from build123d import *

# Parameters (mm, degrees)
F0_R     = 12.5
F1_DEPTH = 25
F2_R     = 7.5
F3_DEPTH = 18
F4_R     = 6.85
F5_DEPTH = 7
F7_DEPTH = 13
F8_SIZE  = 0.5


with BuildPart() as f1:
    # F0 (on Top) → F1 (new body)
    with BuildSketch(Plane.XY):
        Circle(F0_R)
    extrude(amount=F1_DEPTH)

    # F2 (on face) → F3 (cut)
    with BuildSketch(Plane(origin=(0, 0, 0), x_dir=(1, 0, 0), z_dir=(0, 0, -1))):
        Circle(F2_R)
    extrude(amount=-F3_DEPTH, mode=Mode.SUBTRACT)

    # F4 (on face) → F5 (cut)
    with BuildSketch(Plane.XY.offset(25)):
        Circle(F4_R)
    extrude(amount=-F5_DEPTH, mode=Mode.SUBTRACT)

    # F6 (on face) → F7 (cut)
    with BuildSketch(Plane.XY.offset(25)):
        with BuildLine():
            ThreePointArc((-5.9371710435, -11), (-3.0618621785, -12.1191996435), (0, -12.5))
            Line((0, -12.5), (0, -11))
            Line((0, -11), (-5.9371710435, -11))
        make_face()
        with BuildLine():
            Line((0, -11), (0, -12.5))
            ThreePointArc((0, -12.5), (3.0618621785, -12.1191996435), (5.9371710435, -11))
            Line((5.9371710435, -11), (0, -11))
        make_face()
    extrude(amount=-F7_DEPTH, mode=Mode.SUBTRACT)

    # F8
    f8_edges = [f1.edges().sort_by_distance(p)[0] for p in [
        (-12.5, 0, 0),
    ]]
    chamfer(f8_edges, length=F8_SIZE)


solid = f1.part
Can you work these out from the model? Positions are in its coordinate system, mm. A direction names the side the tool comes from. Give positions to 0.01 mm unless a question says otherwise; leave off trailing zeros. Loops run counter-clockwise (first coordinate to the right, second up) from the corner with the lowest first, then second, coordinate; pieces in that order, holes last. Notation, with made-up numbers: (73.25, 8.5) - (96.25, 8.5) arc R9 cw to (96.25, 25.5) - close; hole circle Ø5 at (76, 14.25). An arc over 180 degrees is marked (long way). Return JSON: item names as keys, results as strings.
1. If I drill on line 1 (Y direction, x = 0, z = 21); line 2 (Y direction, x = 0, z = 8.75), over which ranges is the centre line in solid material (lowest first)?
Output values:
{"line 1": "y = -11 to -6.85, 6.85 to 12.5", "line 2": "y = -12.5 to -7.5, 7.5 to 12.5"}
2. For faces 1 (the face through (-6, -5, 0)), 2 (the face through (0, -12, 12)), 3 (the face through (-7.493, -0.33, 8.874)), which set-ups out of +Z, -Z, +X, -X, +Y, -Y let a thin tool reach every point of the face, with its end or its side?
Output values:
{"face 1": "-Z, +X, -X, +Y, -Y", "face 2": "+Z, +X, -X, -Y", "face 3": "-Z"}
3. I'm going to push flat-ended pins straight in: pin 1 Ø10 at (x, z) = (6.5, 21) entering from -Y; pin 2 Ø10 at (x, z) = (-6, 20) entering from +Y; pin 3 Ø4 at (y, z) = (6.5, 11) entering from +X; pin 4 Ø1.5 at (x, y) = (1, 4.5) entering from -Z. Where does each tip first touch, or does it pass through?
Output values:
{"pin 1": "stops at y = -11", "pin 2": "stops at y = 12.46", "pin 3": "stops at x = 11.66", "pin 4": "passes through"}
4. I want a section at D-D on z = 14.5. Please give me the cut outline in (x, y).
Output values:
{"outline": "(-5.94, -11) - (5.94, -11) arc R12.5 ccw (long way) to start; hole circle Ø15 at (0, 0)"}
5. I want a section at B-B on x = 0. Please give me the cut outline in (y, z).
Output values:
{"outline": "(-12.5, 0.5) - (-12, 0) - (-7.5, 0) - (-7.5, 18) - (-6.85, 18) - (-6.85, 25) - (-11, 25) - (-11, 12) - (-12.5, 12) - close; (6.85, 18) - (7.5, 18) - (7.5, 0) - (12, 0) - (12.5, 0.5) - (12.5, 25) - (6.85, 25) - close"}
6. I want a section at C-C on z = 7.5. Please give me the cut outline in (x, y).
Output values:
{"outline": "circle Ø25 at (0, 0); hole circle Ø15 at (0, 0)"}
7. I want a section at A-A on y = 0. Please give me the cut outline in (x, z).
Output values:
{"outline": "(-12.5, 0.5) - (-12, 0) - (-7.5, 0) - (-7.5, 18) - (-6.85, 18) - (-6.85, 25) - (-12.5, 25) - close; (6.85, 18) - (7.5, 18) - (7.5, 0) - (12, 0) - (12.5, 0.5) - (12.5, 25) - (6.85, 25) - close"}
